The listing builds one solid part. Answer for the finished solid, in the listing's coordinates (mm). Face numbers are marked on the shaded views. Give positions to 0.01 mm unless a question says otherwise; leave off trailing zeros. Write each loop counter-clockwise with the first axis right and the second up, starting at its lowest first coordinate (ties: lowest second). Pieces come first, ordered by that corner, then holes. Notation, with made-up numbers: (-10, 22.5) - (31, 22.5) arc R18 cw to (31, 34.5) - close; hole circle Ø8 at (1.5, 53.25). An arc over 180 degrees is marked (long way). Return JSON: item names as keys, results as strings.
from build123d import *

# Parameters (mm, degrees)
SKETCH1_R           = 20
SKETCH1_R_2         = 25
BOSS_EXTRUDE1_DEPTH = 70
SKETCH2_W           = 100
SKETCH2_H           = 94
SKETCH2_W_2         = 140
SKETCH2_H_2         = 90
CUT_EXTRUDE1_DEPTH  = 256.191648227
SKETCH3_W           = 2.284781912
SKETCH3_H           = 94
CUT_EXTRUDE4_DEPTH  = 45
CUT_EXTRUDE5_DEPTH  = 10


with BuildPart() as part:
    # Sketch1 → Boss-Extrude1 (new, symmetric)
    with BuildSketch(Plane.XY):
        with BuildLine():
            Line((172.145187602, 49.918433931), (-175, 40))
            ThreePointArc((-175, 40), (-215, 0), (-175, -40))
            Line((-175, -40), (172.145187602, -49.918433931))
            Line((172.145187602, -49.918433931), (175, -50))
            ThreePointArc((175, -50), (225, 0), (175, 50))
            Line((175, 50), (172.145187602, 49.918433931))
        make_face()
        with Locations((-175, 0)):
            Circle(SKETCH1_R, mode=Mode.SUBTRACT)
        with Locations((175, 0)):
            Circle(SKETCH1_R_2, mode=Mode.SUBTRACT)
    extrude(amount=BOSS_EXTRUDE1_DEPTH, both=True)

    # Sketch2 → Cut-Extrude1 (cut, through all)
    with BuildSketch(Plane(origin=(-1.284665579, 44.963295269, 0), x_dir=(0.9995920864606948, 0.028559773898877126, 0), z_dir=(-0.02855977389887713, 0.9995920864606949, 0))):
        with Locations((-164.928615131, 0)):
            Rectangle(SKETCH2_W, SKETCH2_H)
        with Locations((154.928615131, 0)):
            Rectangle(SKETCH2_W_2, SKETCH2_H_2)
    extrude(amount=-CUT_EXTRUDE1_DEPTH, mode=Mode.SUBTRACT)

    # Sketch3 → Cut-Extrude4 (cut, symmetric)
    with BuildSketch(Plane(origin=(-1.284665579, 44.963295269, 0), x_dir=(0.9995920864606948, 0.02855977389887712, 0), z_dir=(-0.028559773898877122, 0.9995920864606949, 0))):
        with Locations((-174.928615131, 0)):
            Rectangle(SKETCH3_W, SKETCH3_H)
    extrude(amount=CUT_EXTRUDE4_DEPTH, both=True, mode=Mode.SUBTRACT)

    # Sketch4 → Cut-Extrude5 (cut)
    with BuildSketch(Plane.XY.offset(70)):
        with BuildLine():
            Line((-91.281137221, 15), (91.281137221, 15))
            ThreePointArc((91.281137221, 15), (106.281137221, 0), (91.281137221, -15))
            Line((91.281137221, -15), (-91.281137221, -15))
            ThreePointArc((-91.281137221, -15), (-106.281137221, 0), (-91.281137221, 15))
        make_face()
    cut_extrude5 = extrude(amount=-CUT_EXTRUDE5_DEPTH, mode=Mode.SUBTRACT)

    # Mirror1: Cut-Extrude5 across plane
    add(cut_extrude5.mirror(Plane.XY), mode=Mode.SUBTRACT)


solid = part.part
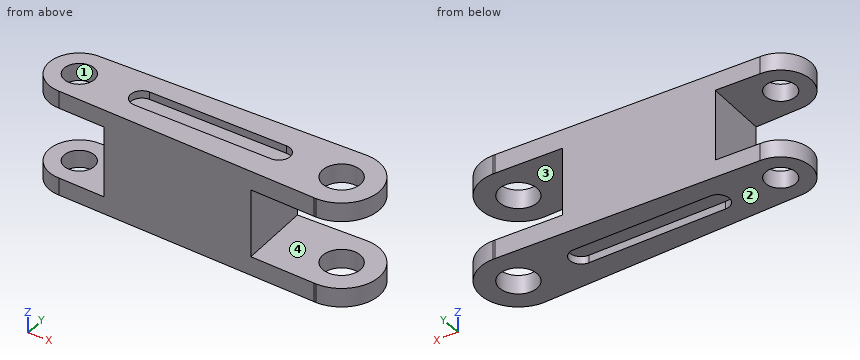
Item 1: Flat-ended cylindrical pins translate along their axes: P1, Ø3, axis at x = -8.5, z = 64.5, coming from the +Y side; P2, Ø1, axis at x = -67, y = 8.5, coming from the +Z side; P3, Ø3, axis at y = 30, z = -16.5, coming from the +X side; P4, Ø24, axis at x = -34, y = -5.5, coming from the -Z side. Find the tip coordinate at first contact, or state that the pin passes through.
Answer below:
{"P1": "stops at y = 44.8", "P2": "stops at z = 60", "P3": "stops at x = 84.15", "P4": "stops at z = -70"}
Item 2: A cutting plane is placed at C-C on x = -70.5. Determine the outline of the cut face in (y, z).
Answer below:
{"outline": "(-42.99, -70) - (-15, -70) - (-15, -60) - (15, -60) - (15, -70) - (42.99, -70) - (42.99, 70) - (15, 70) - (15, 60) - (-15, 60) - (-15, 70) - (-42.99, 70) - close"}
Item 3: The mould has two halves that part along Z. Classify the marked faces 1, 2, 3 and 4: +Z half, -Z half, draft (parallel to the pull), parting line (faces both ways), or undercut.
Answer below:
{"face 1": "draft", "face 2": "-Z half", "face 3": "undercut", "face 4": "undercut"}
Item 4: A cutting plane is placed at B-B on z = 29. Determine the outline of the cut face in (x, y).
Answer below:
{"outline": "(-116.17, 41.68) - (-113.78, -41.75) - (86.32, -47.47) - (83.61, 47.39) - close"}
Item 5: A cutting plane is placed at A-A on x = 138. Determine the outline of the cut face in (y, z).
Answer below:
{"outline": "(-48.94, -70) - (48.94, -70) - (48.94, -45) - (-48.94, -45) - close; (-48.94, 45) - (48.94, 45) - (48.94, 70) - (-48.94, 70) - close"}
Item 6: Consider L1, parallel to Y at x = -175, z = 52; L2, parallel to Z at x = 166, y = 42; L3, parallel to X at y = 0, z = -63.25. Determine where each line is inside the solid, lowest interval first.
Answer below:
{"L1": "y = -40 to -20, 20 to 40", "L2": "z = -70 to -45, 45 to 70", "L3": "x = -215 to -195, -155 to -106.28, 106.28 to 150, 200 to 225"}
Item 7: A cutting plane is placed at D-D on y = 4.5. Give the number of separate pieces and of enclosed holes in the cut face, then the cut area to 3 significant figures.
Answer below:
{"separate pieces": "5", "enclosed holes": "0", "area": "31,100 mm²"}
